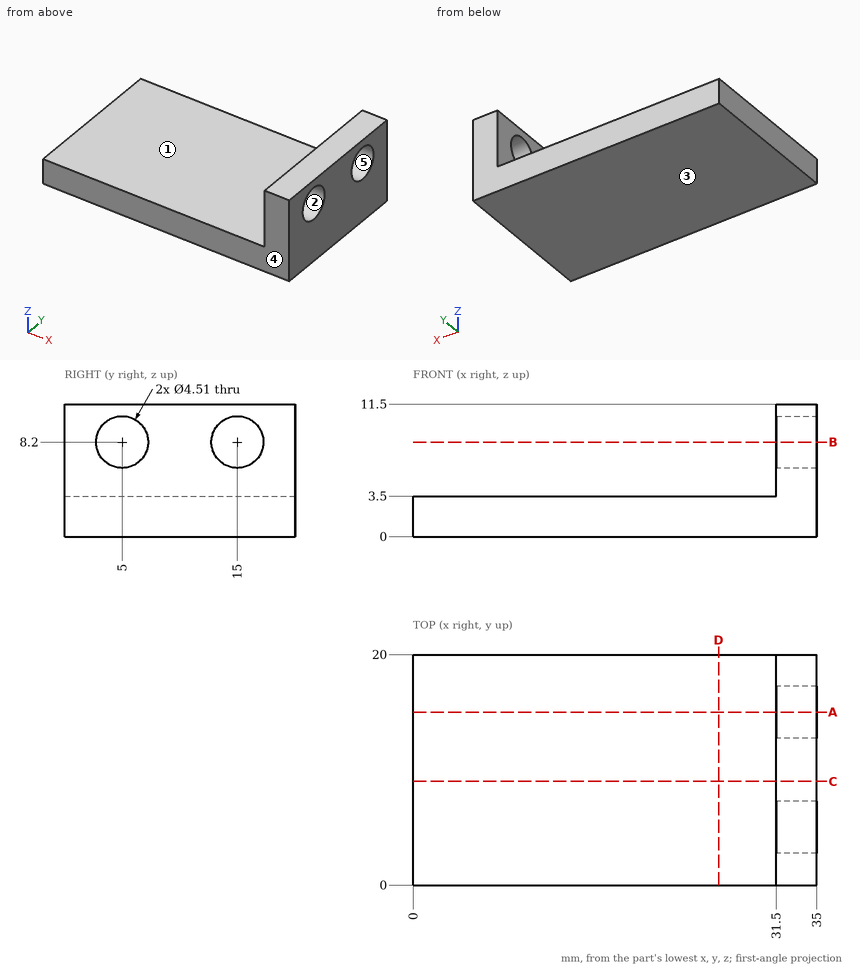
Input: dimensioned drawing with shaded views. Units: mm. Origin: part minimum x, y, z. A direction names the side the tool comes from. Round coordinates to 2 decimals unless told otherwise and drop trailing zeros. Order: outer loops, then holes, each group sorted by start corner. A loop starts at its lowest first (then second) coordinate and runs counter-clockwise, first axis right, second up.
1. Cut plane B-B, the plane z = 8.2. Output: boundary loops of the cut face in (x, y) (3 decimals), then the cut area to 3 significant figures.
The answers:
outline: (31.5, 0) - (35, 0) - (35, 2.745) - (31.5, 2.745) - close; (31.5, 7.255) - (35, 7.255) - (35, 12.745) - (31.5, 12.745) - close; (31.5, 17.255) - (35, 17.255) - (35, 20) - (31.5, 20) - close
area: 38.4 mm2
2. Set-up query: the marked faces 1 and 2. Return all of +Z, -Z, +X, -X, +Y, -Y with unobstructed straight access to the full face (end or side cutting, diameter ignored); none if empty.
The answers:
face 1: +Z, -X, +Y, -Y
face 2: +X, -X
3. Cut plane D-D, the plane x = 26.5. Output: boundary loops of the cut face in (y, z).
The answers:
outline: (0, 0) - (20, 0) - (20, 3.5) - (0, 3.5) - close
4. Mould query, pull axis Z, two halves, no side actions, for the marked faces 3, 4 and 5. Classes: released by +Z, released by -Z, zero draft, split by the parting line, or undercut.
The answers:
face 3: released by -Z
face 4: zero draft
face 5: undercut
5. Cut plane C-C, the plane y = 9. Output: boundary loops of the cut face in (x, z), then the cut area to 4 significant figures.
The answers:
outline: (0, 0) - (35, 0) - (35, 11.5) - (31.5, 11.5) - (31.5, 3.5) - (0, 3.5) - close
area: 150.5 mm2
6. Material intervals for line 1 (Y direction, x = 34.25, z = 8.2) (3 decimals); line 2 (X direction, y = 1.25, z = 6); line 3 (Z direction, x = 15, y = 3.5), sorted ascending.
The answers:
line 1: y = 0 to 2.745, 7.255 to 12.745, 17.255 to 20
line 2: x = 31.5 to 35
line 3: z = 0 to 3.5
7. Pin query (flat end, axial travel): P1, Ø6, axis at x = 18, y = 13, coming from the +Z side; P2, Ø2.5, axis at y = 5, z = 8.2, coming from the +X side; P3, Ø1, axis at x = 18, y = 9.5, coming from the -Z side; P4, Ø2.5, axis at y = 10, z = 6, coming from the -X side. Return the tip coordinate at first contact, or that it passes through.
The answers:
P1: stops at z = 3.5
P2: passes through
P3: stops at z = 0
P4: stops at x = 31.5
8. Cut plane A-A, the plane y = 15. Output: boundary loops of the cut face in (x, z) (3 decimals), then the cut area to 3 significant figures.
The answers:
outline: (0, 0) - (35, 0) - (35, 5.945) - (31.5, 5.945) - (31.5, 3.5) - (0, 3.5) - close; (31.5, 10.455) - (35, 10.455) - (35, 11.5) - (31.5, 11.5) - close
area: 135 mm2
